Source: three-view drawing plus pictorial views. Frame: mm from the lowest corner of the part. A direction names the side the tool comes from. Give positions to 0.01 mm unless a question says otherwise; leave off trailing zeros. Loops run counter-clockwise (first coordinate to the right, second up) from the corner with the lowest first, then second, coordinate; pieces in that order, holes last.
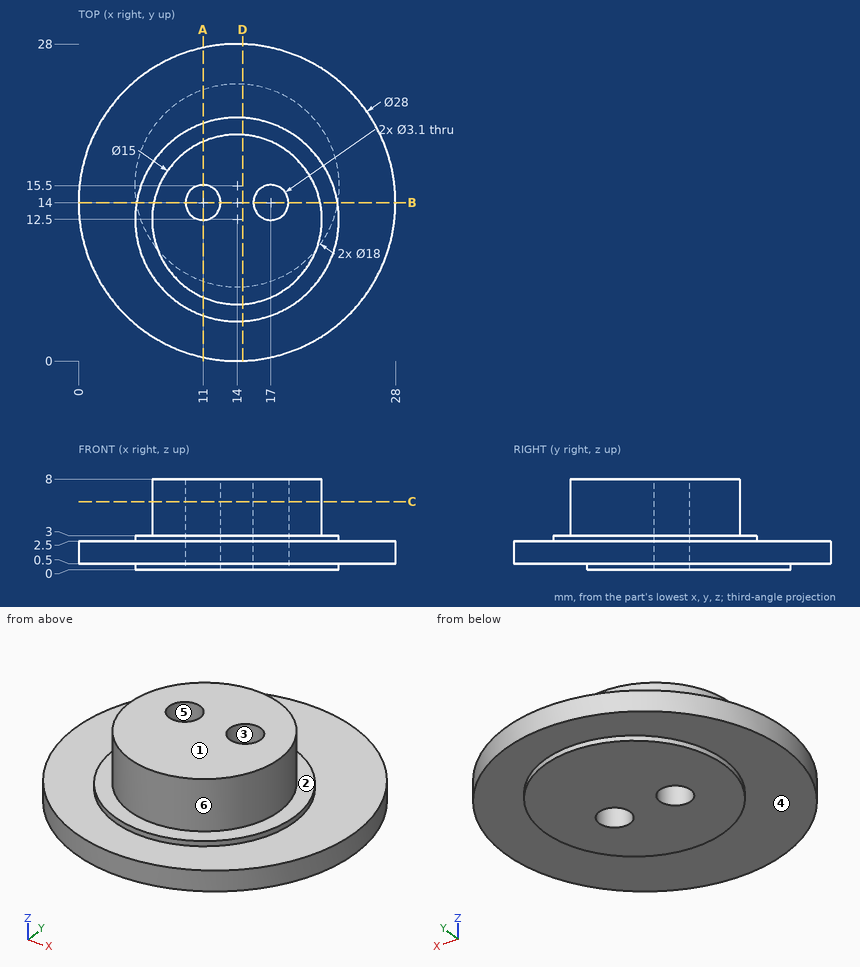
(1) Pin query (flat end, axial travel): pin 1 Ø4 at (x, z) = (14.5, 7) entering from +Y; pin 2 Ø2 at (y, z) = (12.5, 5.5) entering from +X; pin 3 Ø1.5 at (x, z) = (21.5, 6.5) entering from +Y. Return the tip coordinate at first contact, or that it passes through.
Values follow:
pin 1: stops at y = 20
pin 2: stops at x = 21.5
pin 3: stops at y = 15.77
(2) Cut plane D-D (x = 14.5). Return the cut outline in (y, z).
Values follow:
outline: (0.01, 0.5) - (6.51, 0.5) - (6.51, 0) - (24.49, 0) - (24.49, 0.5) - (27.99, 0.5) - (27.99, 2.5) - (21.49, 2.5) - (21.49, 3) - (19.98, 3) - (19.98, 8) - (5.02, 8) - (5.02, 3) - (3.51, 3) - (3.51, 2.5) - (0.01, 2.5) - close
(3) Cut plane A-A (x = 11). Return the cut outline in (y, z).
Values follow:
outline: (0.33, 0.5) - (7.01, 0.5) - (7.01, 0) - (12.45, 0) - (12.45, 8) - (5.63, 8) - (5.63, 3) - (4.01, 3) - (4.01, 2.5) - (0.33, 2.5) - close; (15.55, 0) - (23.99, 0) - (23.99, 0.5) - (27.67, 0.5) - (27.67, 2.5) - (20.99, 2.5) - (20.99, 3) - (19.37, 3) - (19.37, 8) - (15.55, 8) - close
(4) Ray query, probe 1 along Z at (x, y) = (26.75, 15.75); probe 2 along Z at (x, y) = (9, 5.5); probe 3 along Y at (x, z) = (17, 3.25). Return the intervals inside material, ascending.
Values follow:
probe 1: z = 0.5 to 2.5
probe 2: z = 0.5 to 3
probe 3: y = 5.63 to 12.45, 15.55 to 19.37
(5) Cut plane C-C (z = 6). Return the cut outline in (x, y).
Values follow:
outline: circle Ø15 at (14, 12.5); hole circle Ø3.1 at (11, 14); hole circle Ø3.1 at (17, 14)
(6) Cut plane B-B (y = 14). Return the cut outline in (x, z).
Values follow:
outline: (0, 0.5) - (5.13, 0.5) - (5.13, 0) - (9.45, 0) - (9.45, 8) - (6.65, 8) - (6.65, 3) - (5.13, 3) - (5.13, 2.5) - (0, 2.5) - close; (12.55, 0) - (15.45, 0) - (15.45, 8) - (12.55, 8) - close; (18.55, 0) - (22.87, 0) - (22.87, 0.5) - (28, 0.5) - (28, 2.5) - (22.87, 2.5) - (22.87, 3) - (21.35, 3) - (21.35, 8) - (18.55, 8) - close
(7) Reachability of the marked faces 1 and 2 from +Z, -Z, +X, -X, +Y, -Y: full face, straight path, thin tool, end or side. Return the list, or none.
Values follow:
face 1: +Z, +X, -X, +Y, -Y
face 2: +Z
(8) Mould query, pull axis X, two halves, no side actions, for the marked faces 3, 4, 5 and 6. Classes: +X half, -X half, draft (parallel to the pull), parting line (faces both ways), or undercut.
Values follow:
face 3: undercut
face 4: draft
face 5: undercut
face 6: parting line
